from build123d import *

# Parameters (mm, degrees)
F0_R     = 9.525
F1_DEPTH = 101.6
F2_R     = 4.7625
F3_DEPTH = 50.8
F4_R     = 9.525


with BuildPart() as f1:
    # F0 (on Top) → F1 (new body)
    with BuildSketch(Plane.XY):
        Circle(F0_R)
    extrude(amount=F1_DEPTH)

    # F2 (on face) → F3 (cut)
    with BuildSketch(Plane(origin=(0, 0, 0), x_dir=(1, 0, 0), z_dir=(0, 0, -1))):
        Circle(F2_R)
    extrude(amount=-F3_DEPTH, mode=Mode.SUBTRACT)

    # F4
    f4_edges = [f1.edges().sort_by_distance(p)[0] for p in [
        (-9.525, 0, 101.6),
    ]]
    fillet(f4_edges, radius=F4_R)


solid = f1.part
Geometry check sheet. Reference: the model listing, model coordinates, mm. Give positions to 0.01 mm unless a question says otherwise; leave off trailing zeros. Order: outer loops, then holes, each group sorted by start corner. A loop starts at its lowest first (then second) coordinate and runs counter-clockwise, first axis right, second up.
1) Cross-section at D-D (z = 80). Record the boundary of the cut face in (x, y) (3 decimals), then the cut area to 3 significant figures.
Results are:
outline: circle Ø19.05 at (0, 0)
area: 285 mm2
2) Material ranges on probe 1 along Y at (x, z) = (0, 29.5) (1 decimal); probe 2 along Y at (x, z) = (-0.5, 57.5); probe 3 along X at (y, z) = (0.5, 12), recorded low to high.
Results are:
probe 1: y = -9.5 to -4.8, 4.8 to 9.5
probe 2: y = -9.51 to 9.51
probe 3: x = -9.51 to -4.74, 4.74 to 9.51
3) Draft check along Y on faces 1 (the flat face through (-4.4, 2.3, 0)), 2 (the cylindrical face through (-7.559, -5.796, 45.393)), 3 (the cylindrical face through (-3.78, 2.9, 25.04)). Enter one of: released by +Y, released by -Y, zero draft, split by the parting line, or undercut.
Results are:
face 1: zero draft
face 2: split by the parting line
face 3: undercut
4) Gauge pin test, flat ends, axial feed: pin 1 (6 mm diameter, centred on y = -5, z = 86, fed in from -X); pin 2 (10 mm diameter, centred on y = 6.5, z = 56, fed in from -X); pin 3 (1.5 mm diameter, centred on x = 6.5, z = 16.5, fed in from +Y). Record the tip position at first contact, or that the pin passes through.
Results are:
pin 1: stops at x = -9.31
pin 2: stops at x = -9.41
pin 3: stops at y = 7.59
